from build123d import *

# Parameters (mm, degrees)
BOSS_EXTRUDE1_DEPTH = 15
SKETCH1_3_R         = 11
BOSS_EXTRUDE2_DEPTH = 9
CUT_EXTRUDE1_START  = 2
SKETCH1_5_R         = 11
CUT_EXTRUDE1_DEPTH  = 7
FILLET1_R           = 11


with BuildPart() as part:
    # Sketch1 → Boss-Extrude1 (new, symmetric)
    with BuildSketch(Plane.XY):
        with BuildLine():
            ThreePointArc((-162, 18), (-150.581929877, -39.402514855), (-118.066017178, -88.066017178))
            ThreePointArc((-118.066017178, -88.066017178), (-85.539105243, -88.066017178), (-85.539105243, -55.539105243))
            ThreePointArc((-85.539105243, -55.539105243), (-108.083471381, -21.799076966), (-116, 18))
            ThreePointArc((-116, 18), (-139, 41), (-162, 18))
        make_face()
        with BuildLine():
            ThreePointArc((-123, 18), (-139, 34), (-155, 18))
            ThreePointArc((-155, 18), (-144.114773149, -36.723730828), (-113.11626971, -83.11626971))
            ThreePointArc((-113.11626971, -83.11626971), (-90.488852712, -83.11626971), (-90.488852712, -60.488852712))
            ThreePointArc((-90.488852712, -60.488852712), (-114.550628109, -24.477860993), (-123, 18))
        make_face(mode=Mode.SUBTRACT)
    extrude(amount=BOSS_EXTRUDE1_DEPTH, both=True)

    # Sketch1<3> → Boss-Extrude2 (add, symmetric)
    with BuildSketch(Plane.XY):
        with BuildLine():
            ThreePointArc((0, -44), (19.528931575, -39.428680317), (35, -26.664583252))
            Line((35, -26.664583252), (35, 26.664583252))
            ThreePointArc((35, 26.664583252), (19.528931575, 39.428680317), (0, 44))
            Line((0, 44), (-139, 41))
            ThreePointArc((-139, 41), (-125.21351497, 36.410128476), (-116.929481683, 24.472420045))
            Line((-116.929481683, 24.472420045), (-64.032905328, 25.614072772))
            ThreePointArc((-64.032905328, 25.614072772), (-51.356216469, 22.569851157), (-41.818901123, 13.681356252))
            ThreePointArc((-41.818901123, 13.681356252), (-38.072611256, -3.293430459), (-46.023062445, -18.752033163))
            Line((-46.023062445, -18.752033163), (-85.539105243, -55.539105243))
            ThreePointArc((-85.539105243, -55.539105243), (-78.857942833, -70.207416226), (-83.445115781, -85.659119128))
            Line((-83.445115781, -85.659119128), (-55.600860061, -48.770491521))
            ThreePointArc((-55.600860061, -48.770491521), (-51.37310442, -45.258629004), (-46.023062445, -44))
            Line((-46.023062445, -44), (0, -44))
        make_face()
        Circle(SKETCH1_3_R, mode=Mode.SUBTRACT)
    extrude(amount=BOSS_EXTRUDE2_DEPTH, both=True)

    # Sketch1<5> → Cut-Extrude1 (cut)
    # profile 1 of 2: a face of its own
    with BuildSketch(Plane.XY.offset(CUT_EXTRUDE1_START)):
        with BuildLine():
            ThreePointArc((-32, 30.199337741), (-18.292282048, 40.017401433), (-1.898396275, 43.959027419))
            Line((-1.898396275, 43.959027419), (-32, 43.309352518))
            Line((-32, 43.309352518), (-32, 30.199337741))
        make_face()
    # profile 2 of 2: a face of its own
    with BuildSketch(Plane.XY.offset(CUT_EXTRUDE1_START)):
        with BuildLine():
            ThreePointArc((0, -44), (19.528931575, -39.428680317), (35, -26.664583252))
            Line((35, -26.664583252), (35, 26.664583252))
            ThreePointArc((35, 26.664583252), (19.528931575, 39.428680317), (0, 44))
            Line((0, 44), (-1.898396275, 43.959027419))
            ThreePointArc((-1.898396275, 43.959027419), (-18.292282048, 40.017401433), (-32, 30.199337741))
            Line((-32, 30.199337741), (-32, -44))
            Line((-32, -44), (0, -44))
        make_face()
        Circle(SKETCH1_5_R, mode=Mode.SUBTRACT)
    extrude(amount=CUT_EXTRUDE1_DEPTH, mode=Mode.SUBTRACT)

    # Fillet1
    # the kernel refuses this fillet: 11 mm, written as the material it adds along each edge
    with BuildSketch(Plane(origin=(-116.929481683, 24.472420045, -9), x_dir=(0.09199621830017597, -0.9957593563800776, 0), z_dir=(0, 0, 1))) as fillet1_piece_1:
        with BuildLine():
            CenterArc((11.803908742, 10.988267546), FILLET1_R, 175.957949098, 91.395536091)
            Line((0.831270302, 11.763642077), (-0.265993542, 11.841179531))
            Line((-0.265993542, 11.841179531), (-1.097263844, 0.077537453))
            Line((-1.097263844, 0.077537453), (0.211131542, -1.079547809))
            ThreePointArc((0.211131542, -1.079547809), (6.429285778, -0.765233377), (11.245203657, -1.098826755))
            Line((11.245203657, -1.098826755), (11.295995028, 0))
        make_face()
    extrude(amount=18)
    with BuildSketch(Plane(origin=(-85.539105243, -55.539105243, 9), x_dir=(-0.6656229330882777, 0.7462882224361834, 0), z_dir=(0, 0, -1))) as fillet1_piece_2:
        with BuildLine():
            CenterArc((11.236677702, 10.982091478), FILLET1_R, 178.778435739, 94.49143138)
            Line((0.239177665, 11.216597213), (0, 0))
            ThreePointArc((0, 0), (5.932053203, -0.16931694), (11.864106406, 0))
        make_face()
    extrude(amount=18)


solid = part.part
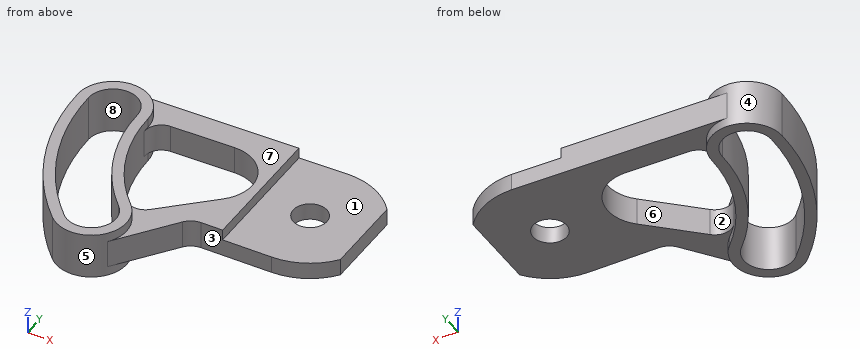
Input: part model. Units: mm. Frame: model coordinates. Face numbers are marked on the shaded views. A direction names the side the tool comes from. Round coordinates to 2 decimals unless told otherwise and drop trailing zeros. Loops run counter-clockwise (first coordinate to the right, second up) from the corner with the lowest first, then second, coordinate; pieces in that order, holes last. Notation, with made-up numbers: (48.25, -17) -> (87.25, -17) arc R19 ccw to (87.25, 16) -> close; hole circle Ø9 at (-30, -26). An arc over 180 degrees is marked (long way). Answer as a JSON object with one key per item and string values. Group by question number.
1) Section query C-C on z = -3.5. Output: boundary loops of the cut face in (x, y), plus the area to 3 significant figures.
2) Section query B-B on y = 0. Output: boundary loops of the cut face in (x, z), plus the area to 3 significant figures.
3) Pin query (flat end, axial travel): pin 1 (3.5 mm diameter, centred on y = 5, z = 6.5, fed in from +X); pin 2 (6 mm diameter, centred on y = -34.5, z = -6.5, fed in from +X); pin 3 (12 mm diameter, centred on x = -40, y = -23, fed in from -Z). Return the tip coordinate at first contact, or that it passes through.
4) Section query D-D on x = 5. Output: boundary loops of the cut face in (y, z).
5) Section query A-A on x = -50.5. Output: boundary loops of the cut face in (y, z), plus the area to 3 significant figures.
6) Ray query, L1, parallel to X at y = -6, z = 5.5; L2, parallel to X at y = -31, z = -6.75; L3, parallel to X at y = -11, z = 12.25. Return the intervals inside material, ascending.
7) Reachability of the marked faces 1, 2, 3 and 4 from +Z, -Z, +X, -X, +Y, -Y: full face, straight path, thin tool, end or side. Return the list, or none.
8) Draft query along X for the marked faces 5, 6, 7 and 8. Return one class per face: +X half, -X half, draft (parallel to the pull), parting line (faces both ways), or undercut.
Reply:
{
 "1": {"outline": "(-162, 18) arc R150 ccw to (-118.07, -88.07) arc R23 ccw to (-83.45, -85.66) -> (-55.6, -48.77) arc R12 cw to (-46.02, -44) -> (0, -44) arc R44 ccw to (35, -26.66) -> (35, 26.66) arc R44 ccw to (0, 44) -> (-139, 41) arc R23 ccw to start; hole (-155, 18) arc R143 ccw to (-113.12, -83.12) arc R16 ccw to (-90.49, -60.49) arc R111 cw to (-123, 18) arc R16 ccw to start; hole (-115.89, 13.22) arc R104 ccw to (-93.44, -46.69) arc R11 ccw to (-77.33, -47.89) -> (-46.02, -18.75) arc R25.62 ccw to (-64.03, 25.61) -> (-105.14, 24.73) arc R11 ccw to start; hole circle Ø22 at (0, 0)", "area": "10,700 mm2"},
 "2": {"outline": "(-160.92, -15) -> (-153.86, -15) -> (-153.86, 15) -> (-160.92, 15) -> close; (-121.53, -15) -> (-114.43, -15) -> (-114.43, 15) -> (-121.53, 15) -> close; (-37.86, -9) -> (-11, -9) -> (-11, 2) -> (-32, 2) -> (-32, 9) -> (-37.86, 9) -> close; (11, -9) -> (35, -9) -> (35, 2) -> (11, 2) -> close", "area": "1,030 mm2"},
 "3": {"pin 1": "stops at x = -32", "pin 2": "stops at x = 30.72", "pin 3": "stops at z = -9"},
 "4": {"outline": "(-43.71, -9) -> (-9.8, -9) -> (-9.8, 2) -> (-43.71, 2) -> close; (9.8, -9) -> (43.71, -9) -> (43.71, 2) -> (9.8, 2) -> close"},
 "5": {"outline": "(-44.87, -9) -> (-22.92, -9) -> (-22.92, 9) -> (-44.87, 9) -> close; (22.09, -9) -> (42.91, -9) -> (42.91, 9) -> (22.09, 9) -> close", "area": "770 mm2"},
 "6": {"L1": "x = -160.07 to -152.97, -120.37 to -113.19, -38.57 to -32", "L2": "x = -153.77 to -146.34, -111.6 to -103.73, -59.18 to 31.22", "L3": "x = -159.17 to -152.03, -119.14 to -111.87"},
 "7": {"face 1": "+Z, +X, +Y, -Y", "face 2": "+Z, -Z", "face 3": "+Z, -Z, +X, -Y", "face 4": "+Y"},
 "8": {"face 5": "parting line", "face 6": "undercut", "face 7": "draft", "face 8": "undercut"}
}
